Study the drawing (mm; zero at the part's minimum x, y, z) and answer. Coordinates: 2 decimals unless noted, no trailing zeros. Order: outer loops, then holes, each group sorted by start corner. A loop starts at its lowest first (then second) coordinate and runs counter-clockwise, first axis right, second up.
1. Find the intervals of material crossed by probe 1 along Y at (x, z) = (17, 0.9); probe 2 along X at (y, z) = (2, 0.4), in increasing order.
2. Determine the mould class of the marked faces 1, 2 and 3 for opening direction X: +X half, -X half, draft (parallel to the pull), parting line (faces both ways), or undercut.
3. The part is cut by section A-A, the plane x = 17. Give the vertices of the cut face in (y, z).
4. A flat-ended cylindrical pin translates along its axis: pin 1 Ø3 at (x, y) = (17, 3) entering from -Z. Find the tip coordinate at first contact, or state that the pin passes through.
5. The part is cut by section B-B, the plane z = 0.4. Give the vertices of the cut face in (x, y).
6. The part is cut by section C-C, the plane y = 3. Give the vertices of the cut face in (x, z), then the cut area to 3 significant figures.
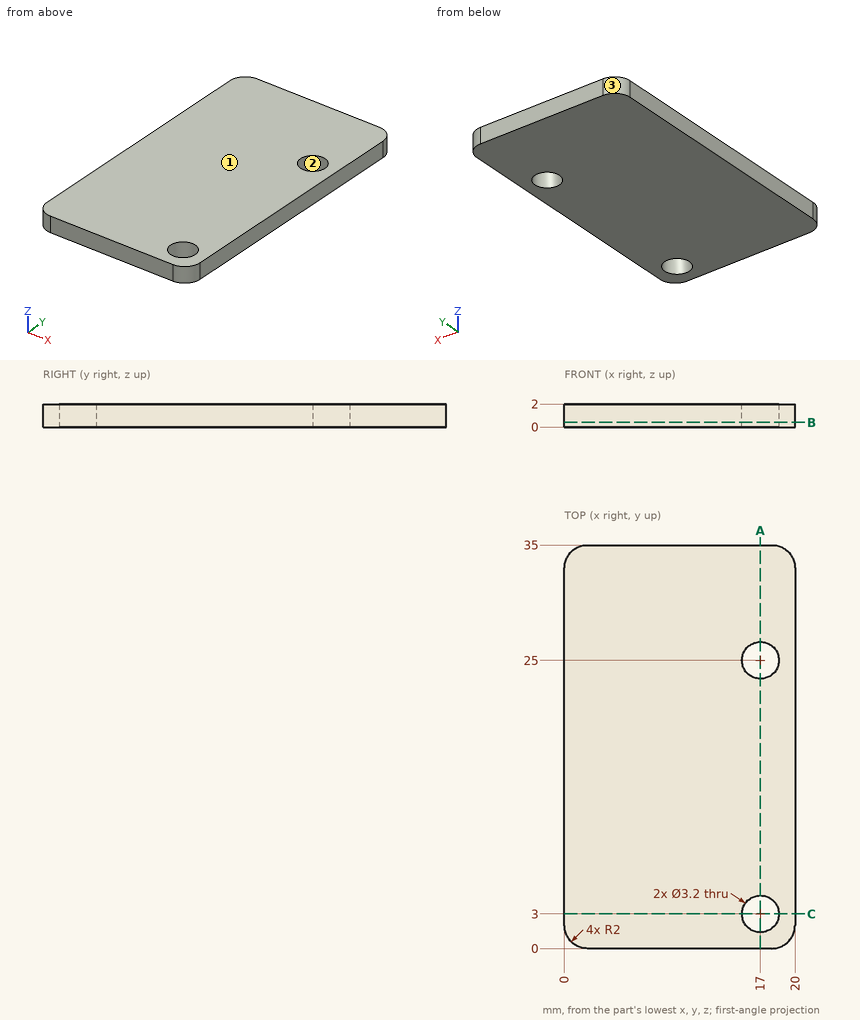
Geometry says:
1. probe 1: y = 0 to 1.4, 4.6 to 23.4, 26.6 to 35
1. probe 2: x = 0 to 15.75, 18.25 to 20
2. face 1: draft
2. face 2: undercut
2. face 3: -X half
3. outline: (0, 0) - (1.4, 0) - (1.4, 2) - (0, 2) - close; (4.6, 0) - (23.4, 0) - (23.4, 2) - (4.6, 2) - close; (26.6, 0) - (35, 0) - (35, 2) - (26.6, 2) - close
4. pin 1: passes through
5. outline: (0, 2) arc R2 ccw to (2, 0) - (18, 0) arc R2 ccw to (20, 2) - (20, 33) arc R2 ccw to (18, 35) - (2, 35) arc R2 ccw to (0, 33) - close; hole circle Ø3.2 at (17, 3); hole circle Ø3.2 at (17, 25)
6. outline: (0, 0) - (15.4, 0) - (15.4, 2) - (0, 2) - close; (18.6, 0) - (20, 0) - (20, 2) - (18.6, 2) - close
6. area: 33.6 mm2
